Build history of the part. All positions in model axes, mm. Coordinates: 2 decimals unless noted, no trailing zeros. Order: outer loops, then holes, each group sorted by start corner. A loop starts at its lowest first (then second) coordinate and runs counter-clockwise, first axis right, second up. Notation, with made-up numbers: (49, 24.25) - (73, 24.25) arc R23 ccw to (73, 57.25) - close; hole circle Ø1 at (-31, 77.25). An arc over 180 degrees is marked (long way). Return JSON: item names as keys, results as strings.
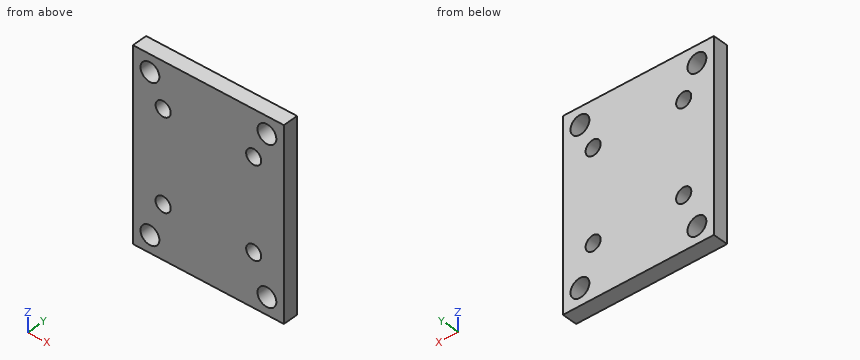
from build123d import *

# Parameters (mm, degrees)
SKETCH1_W           = 25.4
SKETCH1_H           = 31.75
SKETCH1_R           = 1.5875
BOSS_EXTRUDE1_DEPTH = 2.54
SKETCH2_R           = 1.27966848
SKETCH2_R_2         = 1.27
CUT_EXTRUDE1_DEPTH  = 41.739097928


with BuildPart() as part:
    # Sketch1 → Boss-Extrude1 (new body)
    with BuildSketch(Plane(origin=(0, 0, 0), x_dir=(1, 0, 0), z_dir=(0, 1, 0))):
        with Locations((12.7, 15.875)):
            Rectangle(SKETCH1_W, SKETCH1_H)
        with Locations(Location((2.8575, 28.8925, 0), (0, 0, 270))):
            Circle(SKETCH1_R, mode=Mode.SUBTRACT)
        with Locations(Location((22.5425, 28.8925, 0), (0, 0, 270))):
            Circle(SKETCH1_R, mode=Mode.SUBTRACT)
        with Locations(Location((2.8575, 2.8575, 0), (0, 0, 270))):
            Circle(SKETCH1_R, mode=Mode.SUBTRACT)
        with Locations(Location((22.5425, 2.8575, 0), (0, 0, 270))):
            Circle(SKETCH1_R, mode=Mode.SUBTRACT)
    extrude(amount=BOSS_EXTRUDE1_DEPTH)

    # Sketch2 → Cut-Extrude1 (cut, through all)
    with BuildSketch(Plane(origin=(0, 2.54, 0), x_dir=(1, 0, 0), z_dir=(0, 1, 0))):
        with Locations(Location((5.08, 22.86, 0), (0, 0, 270))):
            Circle(SKETCH2_R)
        with Locations(Location((20.32, 22.86, 0), (0, 0, 270))):
            Circle(SKETCH2_R_2)
        with Locations(Location((5.08, 7.62, 0), (0, 0, 270))):
            Circle(SKETCH2_R_2)
        with Locations(Location((20.32, 7.62, 0), (0, 0, 270))):
            Circle(SKETCH2_R_2)
    extrude(amount=-CUT_EXTRUDE1_DEPTH, mode=Mode.SUBTRACT)


solid = part.part
1. Drop a flat-ended pin along its axis: pin 1 (2.5 mm diameter, centred on x = 2.86, z = -28.89, fed in from -Y). Give the stop position or say it passes through.
Check values:
{"pin 1": "through"}
2. Cut at A-A on x = 20.32. Give the cut face in (y, z), plus the area to 3 significant figures.
Check values:
{"outline": "(0, -31.75) - (2.54, -31.75) - (2.54, -24.13) - (0, -24.13) - close; (0, -21.59) - (2.54, -21.59) - (2.54, -8.89) - (0, -8.89) - close; (0, -6.35) - (2.54, -6.35) - (2.54, 0) - (0, 0) - close", "area": "67.7 mm²"}
3. Cut at B-B on z = -7.62. Give the cut face in (x, y), plus the area to 3 significant figures.
Check values:
{"outline": "(0, 0) - (3.81, 0) - (3.81, 2.54) - (0, 2.54) - close; (6.35, 0) - (19.05, 0) - (19.05, 2.54) - (6.35, 2.54) - close; (21.59, 0) - (25.4, 0) - (25.4, 2.54) - (21.59, 2.54) - close", "area": "51.6 mm²"}
4. Probe L1, parallel to X at y = 0.5, z = -7.62; L2, parallel to X at y = 1.1, z = -22.86; L3, parallel to Z at x = 22.25, y = 0.3. List the from-to ranges inside material, lowest first.
Check values:
{"L1": "0 to 3.81, 6.35 to 19.05, 21.59 to 25.4", "L2": "0 to 3.8, 6.36 to 19.05, 21.59 to 25.4", "L3": "-31.75 to -30.45, -27.33 to -4.42, -1.3 to 0"}
5. Cut at C-C on y = 1. State how many separate pieces and enclosed holes the cut face has, plus the area to 3 significant figures.
Check values:
{"separate pieces": "1", "enclosed holes": "8", "area": "754 mm²"}
